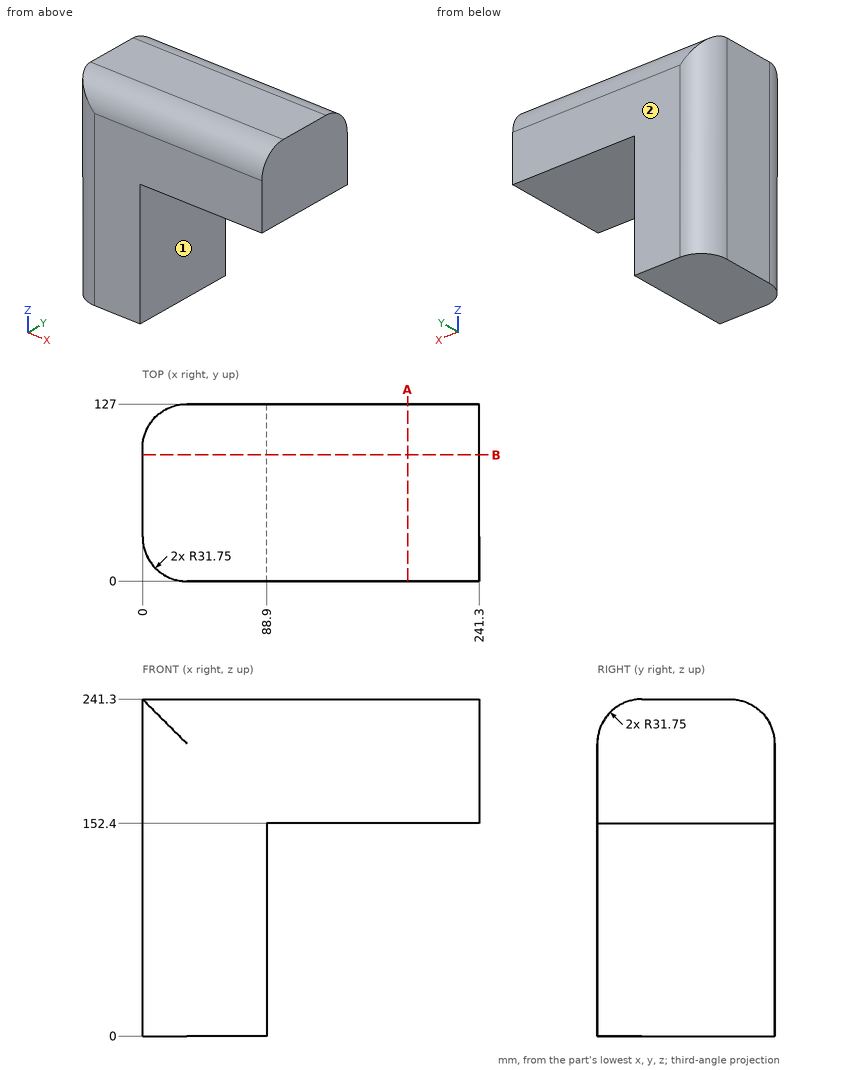
Drawing for the job (mm, zero at the part's lowest x, y, z). A direction names the side the tool comes from. Give positions to 0.01 mm unless a question says otherwise; leave off trailing zeros. Loops run counter-clockwise (first coordinate to the right, second up) from the corner with the lowest first, then second, coordinate; pieces in that order, holes last.
Item 1: Which spindle directions (+Z, -Z, +X, -X, +Y, -Y) get a long thin tool onto all of the face, cutting with end or side? Do the marked faces 1 and 2. Say none if no direction does.
Check values:
face 1: -Z, +X, +Y, -Y
face 2: +Z, -Z, +X, -X, +Y
Item 2: Drop flat-ended pins along their axis: P1, Ø10, axis at y = 17, z = 125.5, coming from the +X side; P2, Ø4, axis at x = 121.5, y = 112.5, coming from the -Z side. Give the stop position or say it passes through.
Check values:
P1: stops at x = 88.9
P2: stops at z = 152.4
Item 3: Slice it at A-A (x = 190). Write the cut outline in (y, z).
Check values:
outline: (0, 152.4) - (127, 152.4) - (127, 209.55) arc R31.75 ccw to (95.25, 241.3) - (31.75, 241.3) arc R31.75 ccw to (0, 209.55) - close
Item 4: Slice it at B-B (y = 90.5). Write the cut outline in (x, z).
Check values:
outline: (0, 0) - (88.9, 0) - (88.9, 152.4) - (241.3, 152.4) - (241.3, 241.3) - (0, 241.3) - close
Item 5: Drill centre lines: line 1 along Z through (x, y) = (133.5, 51); line 2 along X through (y, z) = (94.5, 131.5); line 3 along Z through (x, y) = (20.5, 9.5). Where is each one in solid material? Low to high.
Check values:
line 1: z = 152.4 to 241.3
line 2: x = 0 to 88.9
line 3: z = 0 to 232.2
